```python
from build123d import *

# Parameters (mm, degrees)
SKETCH1_W           = 170
SKETCH1_H           = 90
BOSS_EXTRUDE1_DEPTH = 10
SKETCH2_R           = 1.5
CUT_EXTRUDE1_DEPTH  = 11
FILLET1_R           = 1
SKETCH2_9_R         = 1.5
CUT_EXTRUDE2_DEPTH  = 11
CUT_EXTRUDE3_DEPTH  = 11
FILLET3_R           = 2


with BuildPart() as part:
    # Sketch1 → Boss-Extrude1 (new body)
    with BuildSketch(Plane(origin=(0, 0, 0), x_dir=(1, 0, 0), z_dir=(0, 1, 0))):
        Rectangle(SKETCH1_W, SKETCH1_H)
    extrude(amount=BOSS_EXTRUDE1_DEPTH)

    # Sketch2 → Cut-Extrude1 (cut, through all)
    with BuildSketch(Plane(origin=(0, 10, 0), x_dir=(1, 0, 0), z_dir=(0, 1, 0))):
        with Locations((-74.75, -28)):
            Circle(SKETCH2_R)
        with Locations((-45.25, -28)):
            Circle(SKETCH2_R)
    cut_extrude1 = extrude(amount=-CUT_EXTRUDE1_DEPTH, mode=Mode.SUBTRACT)

    # Mirror1: Cut-Extrude1 across plane
    add(cut_extrude1.mirror(Plane.XY), mode=Mode.SUBTRACT)

    # Fillet1
    fillet1_edges = [part.edges().sort_by_distance(p)[0] for p in [
        (-85, 5, -45),
        (85, 5, -45),
        (85, 5, 45),
        (-85, 5, 45),
    ]]
    fillet(fillet1_edges, radius=FILLET1_R)

    # Sketch2<9> → Cut-Extrude2 (cut, through all)
    with BuildSketch(Plane(origin=(0, 10, 0), x_dir=(1, 0, 0), z_dir=(0, 1, 0))):
        with Locations((67.25, 19)):
            Circle(SKETCH2_9_R)
        with Locations((-7.75, 19)):
            Circle(SKETCH2_9_R)
    extrude(amount=-CUT_EXTRUDE2_DEPTH, mode=Mode.SUBTRACT)

    # Sketch3 → Cut-Extrude3 (cut, through all)
    with BuildSketch(Plane(origin=(0, 10, 0), x_dir=(1, 0, 0), z_dir=(0, 1, 0))):
        Polygon((0, 0), (0, -28), (47.544117112, 0), align=None)
        Polygon((67.25, 0), (19.705882888, -28), (67.25, -28), align=None)
        Polygon((-35.25, -35), (-17.75, -35), (-17.75, 18.828164368), align=None)
        Polygon((-35.25, 35), (-35.25, -18.828164368), (-17.75, 35), align=None)
        Polygon((-74.75, 18), (-74.75, -5.264489844), (-45.25, 18), align=None)
        Polygon((-74.75, -18), (-45.25, -18), (-45.25, 5.264489844), align=None)
    extrude(amount=-CUT_EXTRUDE3_DEPTH, mode=Mode.SUBTRACT)

    # Fillet3
    fillet3_edges = [part.edges().sort_by_distance(p)[0] for p in [
        (-17.75, 5, 35),
        (67.25, 5, 28),
        (-45.25, 5, 18),
        (0, 5, 0),
        (-74.75, 5, -18),
        (-35.25, 5, -35),
    ]]
    fillet(fillet3_edges, radius=FILLET3_R)


solid = part.part
```
Geometry: final body of the model. Coordinates: model frame, mm. Give positions to 0.01 mm unless a question says otherwise; leave off trailing zeros. Loops run counter-clockwise (first coordinate to the right, second up) from the corner with the lowest first, then second, coordinate; pieces in that order, holes last. Notation, with made-up numbers: (23.5, 84.25) -> (36.5, 84.25) arc R28 ccw to (36.5, 107.25) -> close; hole circle Ø10 at (-21.5, 33). An arc over 180 degrees is marked (long way). Use one line per item in the form item = value.
Item 1: Section query A-A on x = 14.5. Output: boundary loops of the cut face in (y, z).
A:
outline = (0, -45) -> (10, -45) -> (10, 0) -> (0, 0) -> close; (0, 19.46) -> (10, 19.46) -> (10, 45) -> (0, 45) -> close
Item 2: Section query B-B on z = 23. Output: boundary loops of the cut face in (x, y), and give its area (3 significant figures).
A:
outline = (-85, 0) -> (-31.35, 0) -> (-31.35, 10) -> (-85, 10) -> close; (-17.75, 0) -> (0, 0) -> (0, 10) -> (-17.75, 10) -> close; (8.49, 0) -> (28.2, 0) -> (28.2, 10) -> (8.49, 10) -> close; (67.25, 0) -> (85, 0) -> (85, 10) -> (67.25, 10) -> close
area = 1,090 mm^2
Item 3: Section query C-C on x = -53. Output: boundary loops of the cut face in (y, z).
A:
outline = (0, -45) -> (10, -45) -> (10, -18) -> (0, -18) -> close; (0, -11.89) -> (10, -11.89) -> (10, 0.85) -> (0, 0.85) -> close; (0, 18) -> (10, 18) -> (10, 45) -> (0, 45) -> close
Item 4: Line query: probe 1 along X at (y, z) = (5.5, -28); probe 2 along Z at (x, y) = (-65, 8); probe 3 along X at (y, z) = (5.75, -1). Output: solid intervals per line, ascending.
A:
probe_1 = -85 to -76.25, -73.25 to -46.75, -43.75 to -35.25, -20.03 to 85
probe_2 = -45 to -18, -2.42 to 10.31, 18 to 45
probe_3 = -85 to -74.75, -66.81 to -50.66, -45.25 to -35.25, -28.8 to -23.55, -17.75 to 85
Item 5: Section query D-D on z = 11.5. Output: boundary loops of the cut face in (x, y).
A:
outline = (-85, 0) -> (-66.51, 0) -> (-66.51, 10) -> (-85, 10) -> close; (-45.25, 0) -> (-35.25, 0) -> (-35.25, 10) -> (-45.25, 10) -> close; (-32.87, 0) -> (-27.61, 0) -> (-27.61, 10) -> (-32.87, 10) -> close; (-17.75, 0) -> (0, 0) -> (0, 10) -> (-17.75, 10) -> close; (28.02, 0) -> (47.72, 0) -> (47.72, 10) -> (28.02, 10) -> close; (67.25, 0) -> (85, 0) -> (85, 10) -> (67.25, 10) -> close
Item 6: Draft query along X for faces 1 (the face through (-85, 5, 1)), 2 (the face through (-17.75, 5, 7)), 3 (the face through (85, 5, 1)). Return one class per face: pulls with the +X half, pulls with the -X half, needs draft (parallel to the pull), parting line crosses it, or undercut.
A:
face_1 = pulls with the -X half
face_2 = undercut
face_3 = pulls with the +X half
